```python
from build123d import *

# Parameters (mm, degrees)
EXTRUDE_1_DEPTH = 50
SKETCH_20_W     = 30
SKETCH_20_H     = 10
EXTRUDE_2_DEPTH = 3
SKETCH_21_W     = 30
SKETCH_21_H     = 10
EXTRUDE_3_DEPTH = 3


with BuildPart() as part:
    # 草图1 → 凸台-拉伸1 (new body)
    with BuildSketch(Plane.XY):
        Polygon((-1.5, -3), (-13, -3), (-13, 3), (-1.5, 3), (-1.5, 5), (-15, 5), (-15, -5), (-1.5, -5), align=None)
        Polygon((-1.5, 3), (-1.5, -3), (-1.5, -5), (1.5, -5), (1.5, -3), (1.5, 3), (1.5, 5), (-1.5, 5), align=None)
        Polygon((1.5, -3), (1.5, -5), (15, -5), (15, 5), (1.5, 5), (1.5, 3), (13, 3), (13, -3), align=None)
    extrude(amount=EXTRUDE_1_DEPTH)

    # 草图20 → 凸台-拉伸2 (add)
    with BuildSketch(Plane(origin=(0, 0, 0), x_dir=(-1, 0, 0), z_dir=(0, 0, -1))):
        Rectangle(SKETCH_20_W, SKETCH_20_H)
    extrude(amount=EXTRUDE_2_DEPTH)

    # 草图21 → 凸台-拉伸3 (add)
    with BuildSketch(Plane.XY.offset(50)):
        Rectangle(SKETCH_21_W, SKETCH_21_H)
    extrude(amount=EXTRUDE_3_DEPTH)


solid = part.part
```
Work out the finished part from the listing and answer in its coordinate system (mm). A direction names the side the tool comes from. Round coordinates to 2 decimals unless told otherwise and drop trailing zeros. Write each loop counter-clockwise with the first axis right and the second up, starting at its lowest first coordinate (ties: lowest second). Pieces come first, ordered by that corner, then holes. Notation, with made-up numbers: (85, 4.5) - (113, 4.5) arc R10 cw to (113, 10.5) - close; hole circle Ø1 at (76, 25.5). An arc over 180 degrees is marked (long way). Return JSON: item names as keys, results as strings. Group by question number.
Q1. The part is cut by section B-B on x = 6.5. Write down the section's boundary in (y, z).
Q2. Find the intervals of material crossed by L1, parallel to X at y = -0.5, z = 8; L2, parallel to Z at x = -3, y = 2.5; L3, parallel to Y at x = -6, z = 32.5, in increasing order.
Q3. For faces 4 (the flat face through (7, 0, 0)), 5 (the flat face through (0, -5, 25)), determine the directions among +Z, -Z, +X, -X, +Y, -Y from which every point of the face is accessible in a straight line to the end or side of a thin tool.
Q4. The part is cut by section C-C on y = -0.5. Write down the section's boundary in (x, z).
Q5. The mould has two halves that part along Z. Classify faces 1 (the flat face through (0, 0, 53)), 2 (the flat face through (-7, 0, 50)), 3 (the flat face through (-15, 0, 25)): released by +Z, released by -Z, zero draft, split by the parting line, or undercut.
Q6. The part is cut by section A-A on z = 21.5. Write down the section's boundary in (x, y), then the cut area to 3 significant figures.
Solved:
{
 "1": {"outline": "(-5, -3) - (5, -3) - (5, 53) - (-5, 53) - close; hole (-3, 0) - (3, 0) - (3, 50) - (-3, 50) - close"},
 "2": {"L1": "-15 to -13, -1.5 to 1.5, 13 to 15", "L2": "-3 to 0, 50 to 53", "L3": "-5 to -3, 3 to 5"},
 "3": {"face 4": "none", "face 5": "+Z, -Z, +X, -X, -Y"},
 "4": {"outline": "(-15, -3) - (15, -3) - (15, 53) - (-15, 53) - close; hole (-13, 0) - (-1.5, 0) - (-1.5, 50) - (-13, 50) - close; hole (1.5, 0) - (13, 0) - (13, 50) - (1.5, 50) - close"},
 "5": {"face 1": "released by +Z", "face 2": "undercut", "face 3": "zero draft"},
 "6": {"outline": "(-15, -5) - (15, -5) - (15, 5) - (-15, 5) - close; hole (-13, -3) - (-1.5, -3) - (-1.5, 3) - (-13, 3) - close; hole (1.5, -3) - (13, -3) - (13, 3) - (1.5, 3) - close", "area": "162 mm²"}
}
